For this review, take the finished solid that the model builds, in its own axes (mm). Face numbers are marked on the shaded views. A direction names the side the tool comes from. Coordinates: 2 decimals unless noted, no trailing zeros. Loops run counter-clockwise (first coordinate to the right, second up) from the corner with the lowest first, then second, coordinate; pieces in that order, holes last. Notation, with made-up numbers: (-13.75, 65) -> (40.25, 65) arc R11 ccw to (40.25, 81) -> close; hole circle Ø3 at (33, 48). An arc over 180 degrees is marked (long way). One line per item, written item: value.
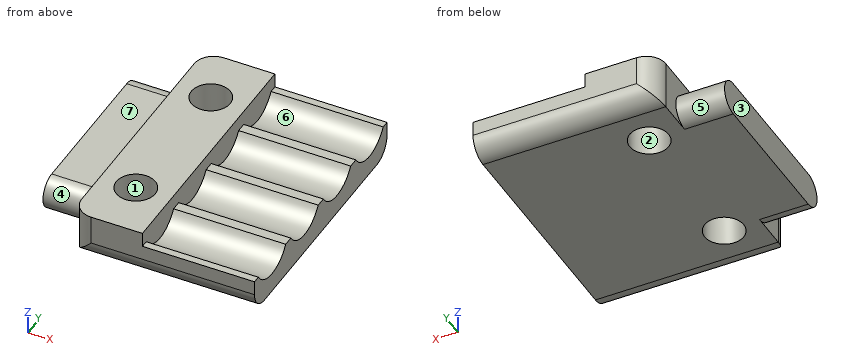
Autodesk Inventor part; units mm, degrees
ref_plane "YZ Plane" through (0, 0, 0) normal (1, 0, 0) x (0, 1, 0)
ref_plane "XZ Plane" through (0, 0, 0) normal (0, 1, 0) x (-1, 0, 0)
ref_plane "XY Plane" through (0, 0, 0) normal (0, 0, 1) x (1, 0, 0)
sketch "スケッチ1" plane through (0, 0, 0) normal (1, 0, 0) x (0, 1, 0)
  arc A0 (-7.5, 1.25) -> (-7.5, -2.75) centre (-7.5, -0.75) ccw construction
  line L0 (-7.5, 1.25) -> (7.5, 1.25) construction
  line L1 (0, 2.5) -> (0, -2.5) construction
  arc A1 (7.5, -2.75) -> (7.5, 1.25) centre (7.5, -0.75) ccw construction
  arc A2 (-7.5, 1) -> (-7.5, -2.5) centre (-7.5, -0.75) ccw
  line L2 (-7.5, 1) -> (7.5, 1)
  line L3 (-7.5, -2.5) -> (7.5, -2.5)
  arc A3 (7.5, -2.5) -> (7.5, 1) centre (7.5, -0.75) ccw
  line L4 (-7.5, -2.75) -> (7.5, -2.75) construction
  line L5 (-13.5, 2.5) -> (13.5, 2.5) construction
  line L6 (13.5, 2.5) -> (13.5, -2.5) construction
  line L7 (13.5, -2.5) -> (-13.5, -2.5) construction
  line L8 (-13.5, -2.5) -> (-13.5, 2.5) construction
  line L9 (-13.5, 2.5) -> (13.5, -2.5) construction
  line L10 (13.5, 2.5) -> (-13.5, -2.5) construction
  line L11 (-13.25, 2.5) -> (13.25, 2.5)
  line L12 (13.25, 2.5) -> (13.25, -2.5)
  line L13 (13.25, -2.5) -> (-13.25, -2.5)
  line L14 (-13.25, -2.5) -> (-13.25, 2.5)
  line L15 (-13.25, 2.5) -> (13.25, -2.5) construction
  line L16 (13.25, 2.5) -> (-13.25, -2.5) construction
  circle A4 centre (-9.75, 2.75) radius 3.25 construction
  circle A5 centre (-3.25, 2.75) radius 3.25 construction
  circle A6 centre (3.25, 2.75) radius 3.25 construction
  circle A7 centre (9.75, 2.75) radius 3.25 construction
  arc A8 (-5.9886, 1) -> (-0.5114, 1) centre (-3.25, 2.75) ccw
  arc A9 (0.5114, 1) -> (5.9886, 1) centre (3.25, 2.75) ccw
  line L17 (-9.75, 2.75) -> (9.75, 2.75) construction
  line L18 (0, 2.5) -> (0, -2.75) construction
  line L19 (-7.0114, 1) -> (-5.9886, 1)
  line L20 (-0.5114, 1) -> (0.5114, 1)
  line L21 (5.9886, 1) -> (7.0114, 1)
  line L22 (-12.4886, 1) -> (-13.25, 1)
  line L23 (12.4886, 1) -> (13.25, 1)
  arc A10 (-12.9904, 2.5) -> (-12.9815, 2.404) centre (-9.75, 2.75) ccw
  arc A11 (-12.4886, 1) -> (-7.0114, 1) centre (-9.75, 2.75) ccw
  arc A12 (7.0114, 1) -> (12.4886, 1) centre (9.75, 2.75) ccw
  arc A13 (12.9815, 2.404) -> (12.9904, 2.5) centre (9.75, 2.75) ccw
  point P0 (0, 0)
  point P1 (0, 0)
  point P2 (0, 0)
  point P3 (-0.0096, 2.5)
  point P4 (0.0096, 2.5)
  point P5 (6.4904, 2.5)
  point P6 (0, 2.75)
  point P7 (-7.5, -2.5)
  point P8 (5.9886, 1)
  point P9 (0.5114, 1)
  point P10 (-0.5114, 1)
  point P11 (-5.9886, 1)
  point P12 (-6.9904, 2.5)
  point P13 (-7.0114, 1)
  point P14 (9.2254, -0.4574)
  point P15 (7.0114, 1)
  point P16 (-7.5, -2.5)
  point P17 (-9.2254, -0.4574)
  point P18 (-7.0114, 1)
  dimension "d0" = 2
  dimension "d1" = 15
  dimension "d2" = 0.25
  dimension "d3" = 6
  dimension "d4" = 6
  dimension "d5" = 0.25
  dimension "d6" = 5
  dimension "d7" = 6.5
  dimension "d8" = 6.5
  dimension "d10" = 6.5
  dimension "d12" = 6.5
  dimension "d27" = 1.5
  dimension "d28" = 2
  dimension "d29" = 0.7614
extrude "押し出し1" add sketch "スケッチ1" against normal blind 33.75 contours L2 A11 A2 | A11 L2 A8 A9 A12 A3 L3 A2 | L2 A8 | A12 L2 A3 | L2 A9
extrude "押し出し2" add sketch "スケッチ1" against normal blind 28.75
extrude "押し出し3" cut sketch "スケッチ1" against normal blind 21.5 contours L2 A11 A2 | A2 A11 L22 L14 L11 L12 L23 A12 A3 L2 | L2 A8 | A12 L2 A3 | L2 A9
extrude "押し出し4" cut sketch "スケッチ1" against normal blind 10
sketch "スケッチ2" plane through (-28.75, -13.25, 2.5) normal (0, 0, 1) x (1, 0, 0)
  line L0 (0, 0) -> (0, 26.5)
  line L1 (18.75, 26.5) -> (0, 26.5)
  line L2 (0, 0) -> (7.25, 0)
  line L3 (7.25, 0) -> (7.25, 26.5)
  line L4 (7.25, 26.5) -> (0, 26.5)
  line L5 (0, 26.5) -> (0, 0)
  line L6 (7.25, 0) -> (7.25, 26.5)
  line L7 (18.75, 0) -> (0, 0)
  line L8 (3.625, 0) -> (3.625, 26.5) construction
  line L9 (18.75, 26.5) -> (0, 26.5)
  circle A0 centre (3.625, 5.75) radius 2
  line L10 (0, 13.25) -> (7.25, 13.25) construction
  circle A1 centre (3.625, 20.75) radius 2
  point P0 (28.75, 13.25)
  point P1 (7.25, 0.2596)
  point P2 (7.25, 7.2404)
  point P3 (7.25, 26.2404)
  dimension "d23" = 4
  dimension "d24" = 15
extrude "押し出し5" cut sketch "スケッチ2" against normal through all contours A0 | A1
fillet "フィレット1" radius 2 4 edges at (-28.75, -13.25, 0) (-28.75, 13.25, 0) (-19.375, 13.25, -2.5) (-19.375, -13.25, -2.5)
equation "\"d5\" = d2"
properties part number "Weight_case_under"
1. For the marked faces 5, 6 and 7, list the 3-axis set-ups (+Z, -Z, +X, -X, +Y, -Y) from which the entire face can be reached by the end or side of a thin tool; tool diameter is ignored.
Return value:
face 5: -X, +Y
face 6: +Z, +X
face 7: +Z, -X, +Y, -Y
2. To check wall thickness, follow probe 1 along Y at (x, z) = (-26.25, 0.25); probe 2 along Y at (x, z) = (-20.5, 0.2); probe 3 along Y at (x, z) = (-16.25, -0.6). State the ranges of each line that lie inside material, in increasing order. Write a range as from..to.
Return value:
probe 1: y = -13.25..-9.15, -5.85..5.85, 9.15..13.25
probe 2: y = -13.25..-11.76, -7.74..-5.26, -1.24..1.24, 5.26..7.74, 11.76..13.25
probe 3: y = -13.25..13.25
3. Take a section at C-C, the plane z = -1.35. Give the boundary of the cut face in (x, y) (3 decimals), and give its area (3 significant figures).
Return value:
outline: (-33.75, -9.144) -> (-28.75, -9.144) -> (-28.75, -11.25) arc R2 ccw to (-27.6, -13.06) -> (-10, -13.06) -> (-10, 13.06) -> (-27.6, 13.06) arc R2 ccw to (-28.75, 11.25) -> (-28.75, 9.144) -> (-33.75, 9.144) -> close; hole circle Ø4 at (-25.125, -7.5); hole circle Ø4 at (-25.125, 7.5)
area: 555 mm2
4. The part is to be moulded in two halves that separate along X. For the marked faces 1, 2, 3 and 4, say which applies: pulls with the +X half, pulls with the -X half, needs draft (parallel to the pull), parting line crosses it, or undercut.
Return value:
face 1: undercut
face 2: undercut
face 3: pulls with the -X half
face 4: needs draft
5. Take a section at A-A, the plane z = 2. Give the boundary of the cut face in (x, y) (3 decimals).
Return value:
outline: (-28.75, -11.25) arc R2 ccw to (-26.75, -13.25) -> (-21.5, -13.25) -> (-21.5, 13.25) -> (-26.75, 13.25) arc R2 ccw to (-28.75, 11.25) -> close; hole circle Ø4 at (-25.125, -7.5); hole circle Ø4 at (-25.125, 7.5)
6. Take a section at B-B, the plane y = -4.25. Give the boundary of the cut face in (x, z).
Return value:
outline: (-33.75, -2.5) -> (-10, -2.5) -> (-10, -0.34) -> (-21.5, -0.34) -> (-21.5, 2.5) -> (-28.75, 2.5) -> (-28.75, 1) -> (-33.75, 1) -> close
7. Take a section at D-D, the plane y = -1.25. Give the boundary of the cut face in (x, z).
Return value:
outline: (-33.75, -2.5) -> (-10, -2.5) -> (-10, 0.19) -> (-21.5, 0.19) -> (-21.5, 2.5) -> (-28.75, 2.5) -> (-28.75, 1) -> (-33.75, 1) -> close
8. Insertion check: pin 1 Ø3 at (x, z) = (-29, 0) entering from -Y; pin 2 Ø0.5 at (x, y) = (-16, 0) entering from +Z; pin 3 Ø2 at (x, z) = (-22.5, -2) entering from -Y. Each pin has a flat end and moves straight along its axis. Give the tip position at first contact, or say it passes through.
Return value:
pin 1: stops at y = -13.1
pin 2: stops at z = 1
pin 3: stops at y = -13.19
